Input: part model. Units: mm. Frame: model coordinates. A direction names the side the tool comes from. Round coordinates to 2 decimals unless told otherwise and drop trailing zeros. Write each loop counter-clockwise with the first axis right and the second up, starting at its lowest first coordinate (ties: lowest second). Pieces come first, ordered by that corner, then holes. Notation, with made-up numbers: (78, 41) - (120, 41) arc R25 cw to (120, 65) - close; hole circle Ø11 at (15.25, 13.25). An arc over 180 degrees is marked (long way). Use one line per item in the form item = value.
```python
from build123d import *

# Parameters (mm, degrees)
SKETCH1_W           = 38
SKETCH1_H           = 21
BOSS_EXTRUDE1_DEPTH = 78
SKETCH2_R           = 4
CUT_EXTRUDE1_DEPTH  = 81.964498393
SKETCH3_R           = 4
BOSS_EXTRUDE2_DEPTH = 140


with BuildPart() as part:
    # Sketch1 → Boss-Extrude1 (new body)
    with BuildSketch(Plane.XY):
        Rectangle(SKETCH1_W, SKETCH1_H)
    extrude(amount=BOSS_EXTRUDE1_DEPTH)

    # Sketch2 → Cut-Extrude1 (cut, through all)
    with BuildSketch(Plane.XY.offset(78)):
        Circle(SKETCH2_R)
    extrude(amount=-CUT_EXTRUDE1_DEPTH, mode=Mode.SUBTRACT)

    # Sketch3 → Boss-Extrude2 (add)
    with BuildSketch(Plane.XY.offset(109)):
        Circle(SKETCH3_R)
    extrude(amount=-BOSS_EXTRUDE2_DEPTH)


solid = part.part
```
(1) Cut plane A-A on x = 0. Output: boundary loops of the cut face in (y, z).
Derived:
outline = (-10.5, 0) - (-4, 0) - (-4, -31) - (4, -31) - (4, 0) - (10.5, 0) - (10.5, 78) - (4, 78) - (4, 109) - (-4, 109) - (-4, 78) - (-10.5, 78) - close
(2) Material intervals for L1, parallel to Z at x = -17, y = -7; L2, parallel to X at y = -0.25, z = -1.5; L3, parallel to Y at x = -1, z = -12, sorted ascending.
Derived:
L1 = 0 to 78
L2 = -3.99 to 3.99
L3 = -3.87 to 3.87
(3) Cut plane C-C on x = 6. Output: boundary loops of the cut face in (y, z), then the cut area to 3 significant figures.
Derived:
outline = (-10.5, 0) - (10.5, 0) - (10.5, 78) - (-10.5, 78) - close
area = 1,640 mm^2
(4) Cut plane B-B on y = 0. Output: boundary loops of the cut face in (x, z).
Derived:
outline = (-19, 0) - (-4, 0) - (-4, -31) - (4, -31) - (4, 0) - (19, 0) - (19, 78) - (4, 78) - (4, 109) - (-4, 109) - (-4, 78) - (-19, 78) - close
(5) Cut plane D-D on y = 7.25. Output: boundary loops of the cut face in (x, z).
Derived:
outline = (-19, 0) - (19, 0) - (19, 78) - (-19, 78) - close
(6) First-contact query: pin 1 Ø5 at (x, y) = (10.5, 0.5) entering from +Z; pin 2 Ø1 at (x, y) = (-8.5, 0) entering from -Z. Flat tips, straight axial feed; report the tip coordinate or a pass-through.
Derived:
pin_1 = 78
pin_2 = 0
(7) Access query for faces 1 (the face through (19, 0, 38)), 2 (the face through (-0.867, -3.905, 93.717)), 3 (the face through (-0.867, -3.905, -15.283)). Directions: +Z, -Z, +X, -X, +Y, -Y. A direction counts if a zero-diameter tool reaches every point of the face in a straight line with its end or side. Return the directions, or none.
Derived:
face_1 = +Z, -Z, +X, +Y, -Y
face_2 = +Z
face_3 = -Z
